```python
from build123d import *

# Parameters (mm, degrees)
DODANIE_WYCI_GNI_CIE1_DEPTH = 80
WYTNIJ_WYCI_GNI_CIE1_DEPTH  = 70


with BuildPart() as part:
    # Szkic1 → Dodanie-wyciągnięcie1 (new body)
    with BuildSketch(Plane.XY):
        with BuildLine():
            Line((-13, -3), (13, -3))
            ThreePointArc((13, -3), (14.414213562, -2.414213562), (15, -1))
            Line((15, -1), (15, 25))
            ThreePointArc((15, 25), (14.414213562, 26.414213562), (13, 27))
            Line((13, 27), (-13, 27))
            ThreePointArc((-13, 27), (-14.414213562, 26.414213562), (-15, 25))
            Line((-15, 25), (-15, -1))
            ThreePointArc((-15, -1), (-14.414213562, -2.414213562), (-13, -3))
        make_face()
        with BuildLine():
            Line((-11, 0), (11, 0))
            ThreePointArc((11, 0), (11.707106781, 0.292893219), (12, 1))
            Line((12, 1), (12, 23))
            ThreePointArc((12, 23), (11.707106781, 23.707106781), (11, 24))
            Line((11, 24), (-11, 24))
            ThreePointArc((-11, 24), (-11.707106781, 23.707106781), (-12, 23))
            Line((-12, 23), (-12, 1))
            ThreePointArc((-12, 1), (-11.707106781, 0.292893219), (-11, 0))
        make_face(mode=Mode.SUBTRACT)
    extrude(amount=DODANIE_WYCI_GNI_CIE1_DEPTH)

    # Szkic2 → Wytnij-wyciągnięcie1 (cut)
    with BuildSketch(Plane.XZ.offset(3)):
        Polygon((-15, 80), (63.522310859, 51.420216122), (63.522310859, 80), align=None)
    extrude(amount=-WYTNIJ_WYCI_GNI_CIE1_DEPTH, mode=Mode.SUBTRACT)


solid = part.part
```
Input: part model. Units: mm. Frame: model coordinates. A direction names the side the tool comes from. Round coordinates to 2 decimals unless told otherwise and drop trailing zeros. Loops run counter-clockwise (first coordinate to the right, second up) from the corner with the lowest first, then second, coordinate; pieces in that order, holes last. Notation, with made-up numbers: (28, 49) -> (47, 49) arc R21 cw to (47, 68) -> close; hole circle Ø1 at (46.25, 36.25). An arc over 180 degrees is marked (long way). Use one line per item in the form item = value. Start each with the question number.
Item 1: Section query C-C on x = -4.5. Return the cut outline in (y, z).
Item 2: Section query B-B on y = 19.5. Return the cut outline in (x, z).
Item 3: Section query A-A on z = 14. Return the cut outline in (x, y).
Item 4: Set-up query: faces 5 (the face through (-14.4, 26.43, 39.44)), 6 (the face through (0, 24, 39)). Return all of +Z, -Z, +X, -X, +Y, -Y with unobstructed straight access to the full face (end or side cutting, diameter ignored); none if empty.
Item 5: Contact query for a flat-ended pin moving along its axis: pin 1 Ø4 at (x, y) = (2.5, 23.5) entering from +Z. Output: stop coordinate, or through.
Item 6: Mould query, pull axis Y, two halves, no side actions, for faces 1 (the face through (-12, 12, 39)), 2 (the face through (0, 27, 39)), 3 (the face through (0, 0, 39)), 4 (the face through (15, 12, 34)). Classes: pulls with the +Y half, pulls with the -Y half, needs draft (parallel to the pull), parting line crosses it, or undercut.
Item 7: Material intervals for L1, parallel to X at y = 14, z = 45; L2, parallel to Y at x = -1.5, z = 45; L3, parallel to Z at x = 12, y = -2, sorted ascending. Write a range as from..to.
Ans:
q1.outline = (-3, 0) -> (0, 0) -> (0, 76.18) -> (-3, 76.18) -> close; (24, 0) -> (27, 0) -> (27, 76.18) -> (24, 76.18) -> close
q2.outline = (-15, 0) -> (-12, 0) -> (-12, 78.91) -> (-15, 80) -> close; (12, 0) -> (15, 0) -> (15, 69.08) -> (12, 70.17) -> close
q3.outline = (-15, -1) arc R2 ccw to (-13, -3) -> (13, -3) arc R2 ccw to (15, -1) -> (15, 25) arc R2 ccw to (13, 27) -> (-13, 27) arc R2 ccw to (-15, 25) -> close; hole (-12, 1) arc R1 ccw to (-11, 0) -> (11, 0) arc R1 ccw to (12, 1) -> (12, 23) arc R1 ccw to (11, 24) -> (-11, 24) arc R1 ccw to (-12, 23) -> close
q4.face_5 = +Z, -Z, -X, +Y
q4.face_6 = +Z, -Z
q5.pin_1 = 74.34
q6.face_1 = undercut
q6.face_2 = pulls with the +Y half
q6.face_3 = undercut
q6.face_4 = needs draft
q7.L1 = -15..-12, 12..15
q7.L2 = -3..0, 24..27
q7.L3 = 0..70.17
